Can you work these out from the model? Positions are in its coordinate system, mm. A direction names the side the tool comes from. Give positions to 0.01 mm unless a question says otherwise; leave off trailing zeros. Order: outer loops, then holes, each group sorted by start corner. A loop starts at its lowest first (then second) coordinate and runs counter-clockwise, first axis right, second up.
Item 1: I'm going to push flat-ended pins straight in: pin 1 Ø1.2 at (x, z) = (10, 3.5) entering from -Y; pin 2 Ø2 at (x, z) = (8.5, 4) entering from +Y; pin 3 Ø1.5 at (x, y) = (10, 2.5) entering from +Z. Where does each tip first touch, or does it pass through?
Item 2: I want a section at C-C, the plane x = 6. Write out the boundary of the cut face in (y, z).
Item 3: I want a section at D-D, the plane z = 4.75. Write out the boundary of the cut face in (x, y), then the cut area to 3 significant figures.
Item 4: I want a section at A-A, the plane x = 9. Write out the boundary of the cut face in (y, z), then the cut area to 3 significant figures.
Item 5: I want a section at B-B, the plane y = 7.65. Write out the boundary of the cut face in (x, z).
Item 6: If I drill on line 1 along Y through (x, z) = (9.25, 5.5); line 2 along Z through (x, y) = (12.75, 3.75); line 3 along Z through (x, y) = (6, 10), over which ranges is the centre line in solid material (lowest first)?
Item 7: Which directions (+Z, -Z, +X, -X, +Y, -Y) give clear straight access to the entire face, cutting with the end or side of a thin tool? Please do faces 1 (the flat face through (7, 8, 5.7)), 2 (the flat face through (9, 10.8, 4)), 3 (the flat face through (9, 4.5, 4)), 4 (the flat face through (13, 8, 4)), 5 (the flat face through (5, 8, 4)).
Autodesk Inventor part; units mm, degrees
ref_plane "YZ Plane" through (0, 0, 0) normal (1, 0, 0) x (0, 1, 0)
ref_plane "XZ Plane" through (0, 0, 0) normal (0, 1, 0) x (-1, 0, 0)
ref_plane "XY Plane" through (0, 0, 0) normal (0, 0, 1) x (1, 0, 0)
sketch "Sketch1" plane through (0, 0, 0) normal (0, 0, 1) x (1, 0, 0)
  line L0 (0, 0) -> (18, 0)
  line L1 (18, 0) -> (18, 13)
  line L2 (18, 13) -> (0, 13)
  line L3 (0, 13) -> (0, 0)
  dimension "d0" = 18
  dimension "d1" = 13
extrude "Extrusion1" add sketch "Sketch1" along normal blind 1.7
sketch "Sketch2" plane through (0, 0, 1.7) normal (0, 0, 1) x (1, 0, 0)
  line L0 (5, 10.8) -> (13, 10.8)
  line L1 (13, 10.8) -> (13, 4.5)
  line L2 (13, 4.5) -> (5, 4.5)
  line L3 (5, 4.5) -> (5, 10.8)
  line L4 (0, 13) -> (0, 0)
  line L5 (18, 13) -> (0, 13)
  dimension "d4" = 8
  dimension "d5" = 6.3
  dimension "d6" = 5
  dimension "d7" = 2.2
extrude "Extrusion2" add sketch "Sketch2" along normal blind 4
sketch "Sketch3" plane through (0, 0, 5.7) normal (0, 0, 1) x (1, 0, 0)
  circle A0 centre (9, 7.65) radius 1.75
  line L0 (5, 10.8) -> (5, 4.5)
  line L1 (13, 10.8) -> (5, 10.8)
  point P0 (0, 0)
  dimension "d10" = 3.5
  dimension "d11" = 4
  dimension "d12" = 3.15
extrude "Extrusion3" add sketch "Sketch3" along normal blind 6
properties part number "Switch"
Results list:
1. pin 1: stops at y = 4.5
1. pin 2: stops at y = 10.8
1. pin 3: stops at z = 1.7
2. outline: (0, 0) - (13, 0) - (13, 1.7) - (10.8, 1.7) - (10.8, 5.7) - (4.5, 5.7) - (4.5, 1.7) - (0, 1.7) - close
3. outline: (5, 4.5) - (13, 4.5) - (13, 10.8) - (5, 10.8) - close
3. area: 50.4 mm2
4. outline: (0, 0) - (13, 0) - (13, 1.7) - (10.8, 1.7) - (10.8, 5.7) - (9.4, 5.7) - (9.4, 11.7) - (5.9, 11.7) - (5.9, 5.7) - (4.5, 5.7) - (4.5, 1.7) - (0, 1.7) - close
4. area: 68.3 mm2
5. outline: (0, 0) - (18, 0) - (18, 1.7) - (13, 1.7) - (13, 5.7) - (10.75, 5.7) - (10.75, 11.7) - (7.25, 11.7) - (7.25, 5.7) - (5, 5.7) - (5, 1.7) - (0, 1.7) - close
6. line 1: y = 4.5 to 10.8
6. line 2: z = 0 to 1.7
6. line 3: z = 0 to 5.7
7. face 1: +Z
7. face 2: +Z, +X, -X, +Y
7. face 3: +Z, +X, -X, -Y
7. face 4: +Z, +X, +Y, -Y
7. face 5: +Z, -X, +Y, -Y
